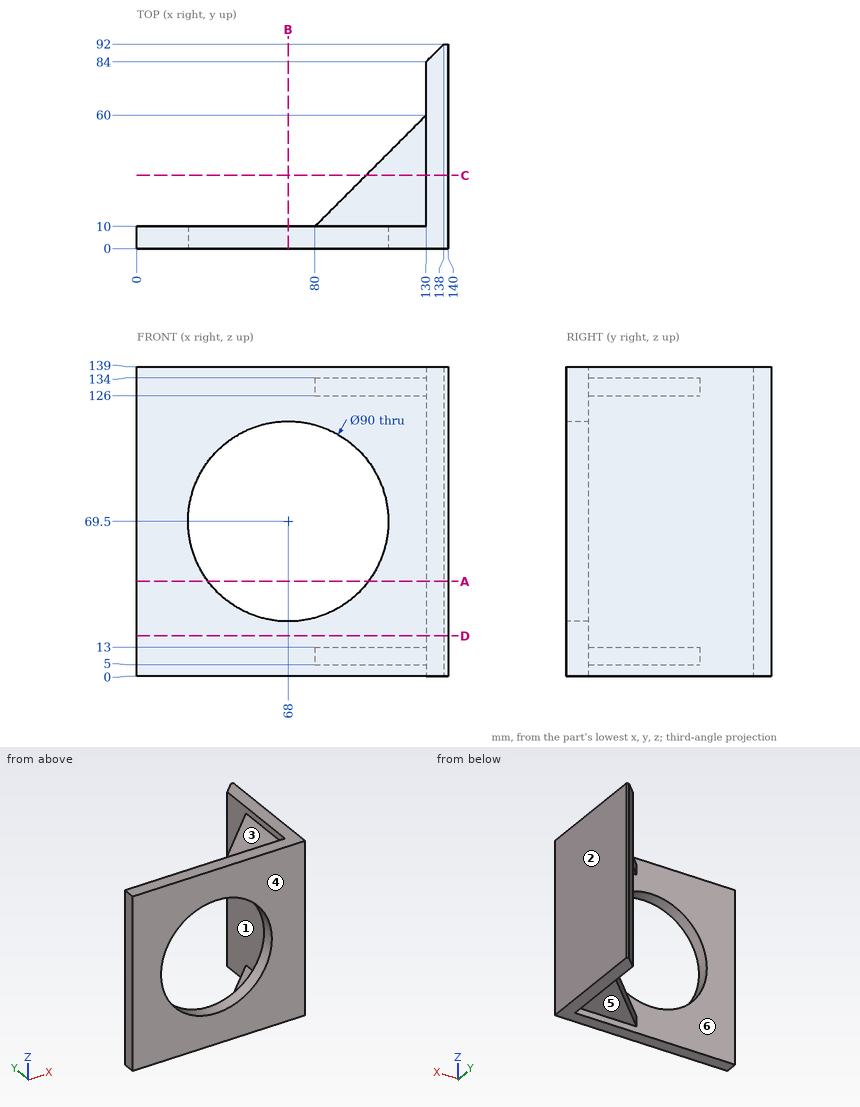
Answer from the drawing. Dimensions are ordinates in mm from the lowest x, y and z of the part. A direction names the side the tool comes from. Round coordinates to 2 decimals unless told otherwise and drop trailing zeros. Loops run counter-clockwise (first coordinate to the right, second up) from the corner with the lowest first, then second, coordinate; pieces in that order, holes last.
Q1. Section B-B on x = 68 is taken. Write down the section's boundary in (y, z), and give its area (3 significant figures).
Q2. Each of these flat-tipped pins is pushed along its axis until it touches: pin 1 (15 mm diameter, centred on x = 110.5, y = 45, fed in from +Z); pin 2 (4 mm diameter, centred on y = 24.5, z = 83, fed in from -X); pin 3 (6 mm diameter, centred on x = 47.5, z = 16, fed in from +Y). Where does it stop, or does it pass through?
Q3. Section C-C on y = 33 is taken. Write down the section's boundary in (x, z), and give its area (3 significant figures).
Q4. Consider probe 1 along X at (y, z) = (8, 69); probe 2 along Z at (x, y) = (96, 16); probe 3 along Y at (x, z) = (50, 15). Determine where each line is inside the solid, lowest interval first.
Q5. Section A-A on z = 42.5 is taken. Write down the section's boundary in (x, y).
Q6. Section D-D on z = 18 is taken. Write down the section's boundary in (x, y), and give its area (3 significant figures).
Q7. Determine the mould class of the marked faces 4, 5 and 6 for opening direction Z: released by +Z, released by -Z, zero draft, split by the parting line, or undercut.
Q8. Which of the six approach directions +Z, -Z, +X, -X, +Y, -Y give full straight-line access (tool end or side, diameter ignored) to the marked faces 1, 2 and 3?
Output:
1. outline: (0, 0) - (10, 0) - (10, 24.5) - (0, 24.5) - close; (0, 114.5) - (10, 114.5) - (10, 139) - (0, 139) - close
1. area: 490 mm2
2. pin 1: stops at z = 134
2. pin 2: stops at x = 130
2. pin 3: stops at y = 10
3. outline: (103, 5) - (130, 5) - (130, 0) - (140, 0) - (140, 139) - (130, 139) - (130, 134) - (103, 134) - (103, 126) - (130, 126) - (130, 13) - (103, 13) - close
3. area: 1,820 mm2
4. probe 1: x = 0 to 23, 113 to 140
4. probe 2: z = 5 to 13, 126 to 134
4. probe 3: y = 0 to 10
5. outline: (0, 0) - (32, 0) - (32, 10) - (0, 10) - close; (104, 0) - (140, 0) - (140, 92) - (138, 92) - (130, 84) - (130, 10) - (104, 10) - close
6. outline: (0, 0) - (140, 0) - (140, 92) - (138, 92) - (130, 84) - (130, 10) - (0, 10) - close
6. area: 2,190 mm2
7. face 4: zero draft
7. face 5: released by -Z
7. face 6: undercut
8. face 1: -X, +Y
8. face 2: +Z, -Z, +X, +Y, -Y
8. face 3: +Z, -X, +Y
